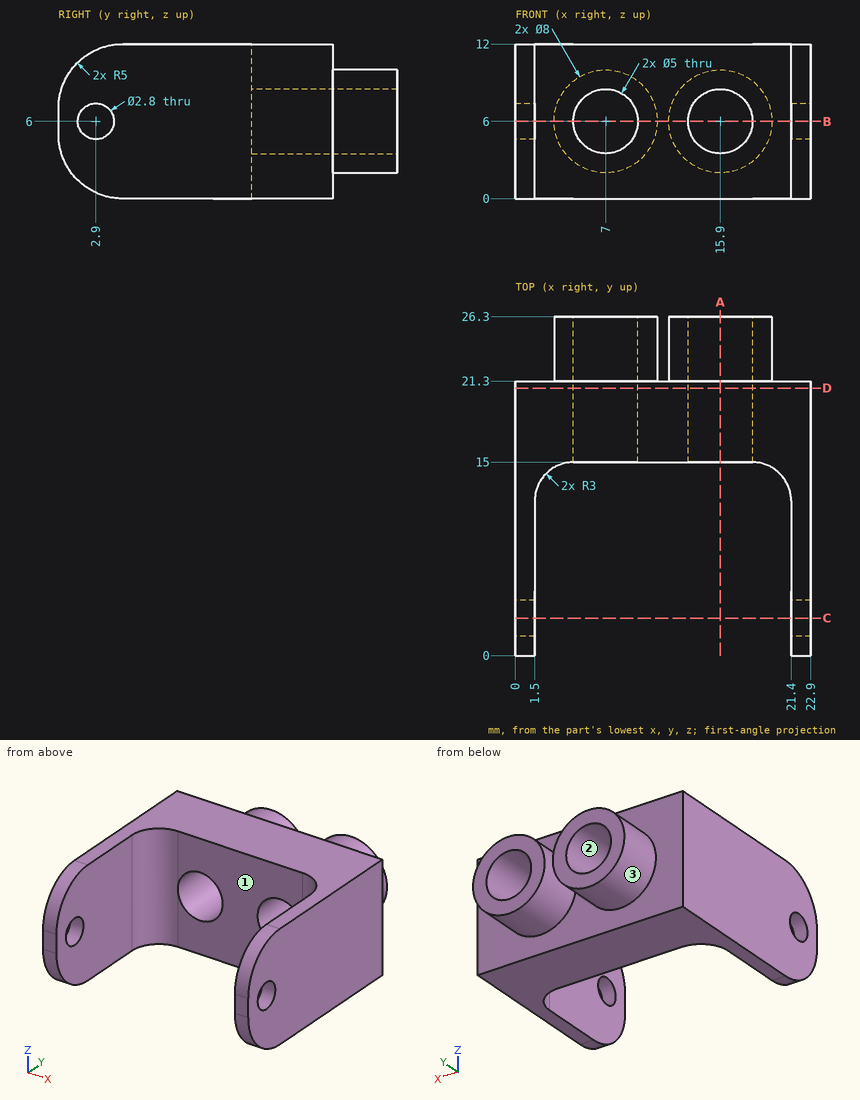
Can you work these out from the drawing? Everything is in mm from the part's minimum corner. A direction names the side the tool comes from. Round coordinates to 2 decimals unless told otherwise and drop trailing zeros. Loops run counter-clockwise (first coordinate to the right, second up) from the corner with the lowest first, then second, coordinate; pieces in that order, holes last. Notation, with made-up numbers: M -11,89 L -3,89 A17 cw -3,121 Z; hole C 36,58.25 d10. An arc over 180 degrees is marked long. Write item = value, one per line.
1. I want a section at A-A, the plane x = 15.9. Write out the boundary of the cut face in (y, z).
Results below:
outline = M 15,0 L 21.3,0 L 21.3,2 L 26.3,2 L 26.3,3.5 L 15,3.5 Z; M 15,8.5 L 26.3,8.5 L 26.3,10 L 21.3,10 L 21.3,12 L 15,12 Z
2. I want a section at D-D, the plane y = 20.75. Write out the boundary of the cut face in (x, z).
Results below:
outline = M 0,0 L 22.9,0 L 22.9,12 L 0,12 Z; hole C 7,6 d5; hole C 15.9,6 d5
3. I want a section at C-C, the plane y = 2.9. Write out the boundary of the cut face in (x, z).
Results below:
outline = M 0,0.46 L 1.5,0.46 L 1.5,4.6 L 0,4.6 Z; M 0,7.4 L 1.5,7.4 L 1.5,11.54 L 0,11.54 Z; M 21.4,0.46 L 22.9,0.46 L 22.9,4.6 L 21.4,4.6 Z; M 21.4,7.4 L 22.9,7.4 L 22.9,11.54 L 21.4,11.54 Z
4. I need wall thicknesses on probe 1 along X at (y, z) = (5.5, 4.25); probe 2 along X at (y, z) = (19.5, 6); probe 3 along Y at (x, z) = (7.25, 9.75). Which ranges of each line are inside material? Lowest first, please.
Results below:
probe_1 = 0 to 1.5, 21.4 to 22.9
probe_2 = 0 to 4.5, 9.5 to 13.4, 18.4 to 22.9
probe_3 = 15 to 26.3
5. Will these pins go through, and if not, where does the flat tip stop? P1, Ø6, axis at x = 13.5, z = 4.5, coming from the -Y side; P2, Ø1, axis at y = 22, z = 4.5, coming from the +X side; P3, Ø1, axis at x = 19.5, z = 2, coming from the -Y side.
Results below:
P1 = 15
P2 = 19.77
P3 = 14.54
6. Which directions (+Z, -Z, +X, -X, +Y, -Y) give clear straight access to the entire face, cutting with the end or side of a thin tool? Please do the marked faces 1, 2 and 3.
Results below:
face_1 = +Z, -Z, -Y
face_2 = +Y, -Y
face_3 = +Y
7. I want a section at B-B, the plane z = 6. Count the separate pieces of the cut face and the enclosed holes in it, and give its area (3 significant figures).
Results below:
separate_pieces = 5
enclosed_holes = 0
area = 152 mm²
